```python
from build123d import *

# Parameters (mm, degrees)
F0_W     = 40
F0_H     = 100
F1_DEPTH = 3
F4_D     = 3
F7_DEPTH = 41.597918


with BuildPart() as f1:
    # F0 (on Top) → F1 (new body)
    with BuildSketch(Plane.XY):
        with Locations((20, 50)):
            Rectangle(F0_W, F0_H)
    extrude(amount=F1_DEPTH)

    # F4 (through all)
    with Locations(Plane.XY.offset(3)):
        with Locations((20, 50), (20, 25)):
            Hole(F4_D / 2)

    # F6 (on face) → F7 (cut)
    with BuildSketch(Plane.XY.offset(3)):
        with BuildLine():
            ThreePointArc((27.516141, 19.716375), (30.283625, 17.516141), (32.483859, 20.283625))
            Line((32.483859, 20.283625), (27.945864, 60.025373))
            ThreePointArc((27.945864, 60.025373), (25.17838, 62.225608), (22.978145, 59.458124))
            Line((22.978145, 59.458124), (27.516141, 19.716375))
        make_face()
    extrude(amount=-F7_DEPTH, mode=Mode.SUBTRACT)

    # F8: F1 across plane


with BuildPart() as f1_1:
    add(f1.part)
    add(f1.part.mirror(Plane.YZ))


solid = f1_1.part
```
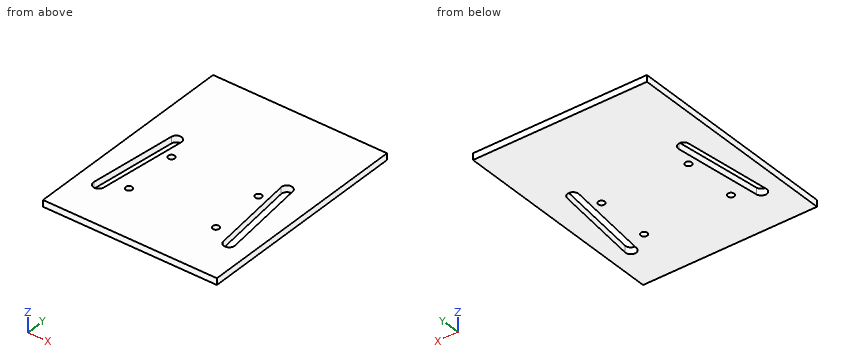
Verification items for the finished model (mm, model axes). Coordinates: 2 decimals unless noted, no trailing zeros. Loops run counter-clockwise (first coordinate to the right, second up) from the corner with the lowest first, then second, coordinate; pieces in that order, holes last. Notation, with made-up numbers: (-21.5, 89.25) - (12.5, 89.25) arc R17 ccw to (12.5, 101.25) - close; hole circle Ø6 at (-22.5, 77.5). An arc over 180 degrees is marked (long way). Put each result on its own line as item: value.
Item 1: Section check A-A (z = 0.75). Enter the section's corners in (x, y).
Conclusion:
outline: (-40, 0) - (40, 0) - (40, 100) - (-40, 100) - close; hole (-32.48, 20.28) arc R2.5 ccw to (-27.52, 19.72) - (-22.98, 59.46) arc R2.5 ccw to (-27.95, 60.03) - close; hole circle Ø3 at (-20, 25); hole circle Ø3 at (-20, 50); hole circle Ø3 at (20, 25); hole circle Ø3 at (20, 50); hole (22.98, 59.46) - (27.52, 19.72) arc R2.5 ccw to (32.48, 20.28) - (27.95, 60.03) arc R2.5 ccw to start
Item 2: Gauge pin test, flat end, axial feed: pin 1 Ø2.5 at (x, y) = (20, 50) entering from -Z. Record the tip position at first contact, or that the pin passes through.
Conclusion:
pin 1: passes through
Item 3: Section check C-C (y = 50). Enter the section's corners in (x, z), then the cut area to 3 significant figures.
Conclusion:
outline: (-40, 0) - (-29.09, 0) - (-29.09, 3) - (-40, 3) - close; (-24.06, 0) - (-21.5, 0) - (-21.5, 3) - (-24.06, 3) - close; (-18.5, 0) - (18.5, 0) - (18.5, 3) - (-18.5, 3) - close; (21.5, 0) - (24.06, 0) - (24.06, 3) - (21.5, 3) - close; (29.09, 0) - (40, 0) - (40, 3) - (29.09, 3) - close
area: 192 mm2
Item 4: Section check B-B (x = -20). Enter the section's corners in (y, z).
Conclusion:
outline: (0, 0) - (23.5, 0) - (23.5, 3) - (0, 3) - close; (26.5, 0) - (48.5, 0) - (48.5, 3) - (26.5, 3) - close; (51.5, 0) - (100, 0) - (100, 3) - (51.5, 3) - close
Item 5: Scan lines: line 1 along Y through (x, z) = (-20, 2); line 2 along Y through (x, z) = (19.5, 2.1); line 3 along X through (y, z) = (57.5, 1.15). Record each from-to range of solid material in increasing order.
Conclusion:
line 1: y = 0 to 23.5, 26.5 to 48.5, 51.5 to 100
line 2: y = 0 to 23.59, 26.41 to 48.59, 51.41 to 100
line 3: x = -40 to -28.23, -23.2 to 23.2, 28.23 to 40
Item 6: Section check D-D (x = 29.5). Enter the section's corners in (y, z).
Conclusion:
outline: (0, 0) - (17.55, 0) - (17.55, 3) - (0, 3) - close; (46.41, 0) - (100, 0) - (100, 3) - (46.41, 3) - close
